Can you work these out from the model? Positions are in its coordinate system, mm. Round coordinates to 2 decimals unless told otherwise and drop trailing zeros. Loops run counter-clockwise (first coordinate to the right, second up) from the corner with the lowest first, then second, coordinate; pieces in that order, holes last.
(1) If I drill on line 1 along Z through (x, y) = (0, 0.3); line 2 along Y through (x, z) = (-25.5, 29), over which ranges is the centre line in solid material (lowest first)?
(2) I want a section at D-D on y = 10.75. Give the number of separate pieces and of enclosed holes in the cut face, plus the area to 3 significant figures.
(3) I want a section at C-C on y = 2.25. Write out the boundary of the cut face in (x, z), plus the area to 3 significant figures.
(4) I want a section at B-B on x = -6. Write out the boundary of the cut face in (y, z).
(5) Will these pins go through, and if not, where does the flat tip stop? pin 1 Ø0.8 at (x, z) = (33.5, 19) entering from +Y; pin 2 Ø4 at (x, y) = (30, 10) entering from -Z; pin 3 Ø11.5 at (x, z) = (27, -18.5) entering from +Y.
(6) I want a section at A-A on z = 0. Write out the boundary of the cut face in (x, y), plus the area to 3 significant figures.
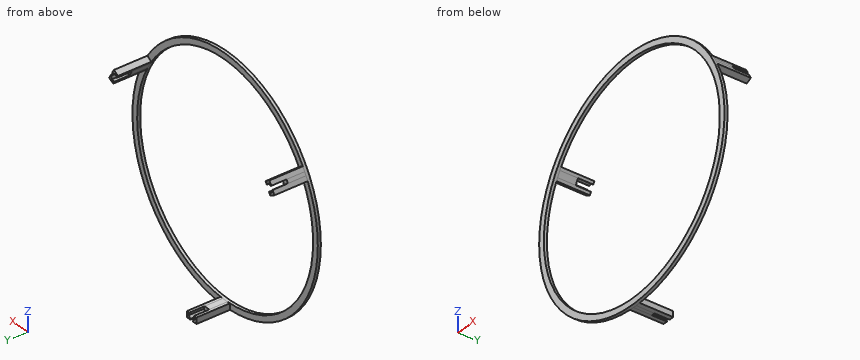
Autodesk Inventor part; units mm, degrees
ref_plane "YZ Plane" through (0, 0, 0) normal (1, 0, 0) x (0, 1, 0)
ref_plane "XZ Plane" through (0, 0, 0) normal (0, 1, 0) x (-1, 0, 0)
ref_plane "XY Plane" through (0, 0, 0) normal (0, 0, 1) x (1, 0, 0)
sketch "Sketch1" plane through (0, 0, 0) normal (0, 1, 0) x (-1, 0, 0)
  circle A0 centre (0, 0) radius 39.5
  circle A1 centre (0, 0) radius 37.5
  dimension "d0" = 79
  dimension "d1" = 75
extrude "Extrusion1" add sketch "Sketch1" along normal blind 1
sketch "Sketch2" plane through (0, 1, 0) normal (0, 1, 0) x (1, 0, 0)
  circle A0 centre (0, 0) radius 37.5
  circle A1 centre (0, 0) radius 39.5
  line L0 (0, 39.5) -> (0, 37.5) construction
  line L1 (-0.57, 39.24) -> (0, 39.24)
  line L2 (-1.31, 38.5) -> (-1.31, 38.5)
  line L3 (-1.31, 38.5) -> (-1.31, 38.49)
  line L4 (-1.2707, 37.74) -> (0, 37.74)
  line L5 (-0.57, 39.24) -> (-1.31, 38.5)
  line L6 (-1.31, 38.49) -> (-1.2707, 37.74)
  line L7 (0, 0) -> (2.0673, 39.4459) construction
  line L8 (0, 0) -> (-2.0673, 39.4459) construction
  line L9 (1.9626, 37.4486) -> (2.0673, 39.4459)
  line L10 (-1.9626, 37.4486) -> (-2.0673, 39.4459)
  line L11 (-1, 37.74) -> (-1, 37.4867)
  line L12 (0.57, 39.24) -> (0, 39.24)
  line L13 (1.31, 38.5) -> (1.31, 38.5)
  line L14 (1.31, 38.5) -> (1.31, 38.49)
  line L15 (1.2707, 37.74) -> (0, 37.74)
  line L16 (0.57, 39.24) -> (1.31, 38.5)
  line L17 (1.31, 38.49) -> (1.2707, 37.74)
  line L18 (-0.57, 39.24) -> (-0.57, 39.4959)
  line L19 (-0.57, 39.4959) -> (-2.0673, 39.4459)
  line L20 (-1, 37.4867) -> (-1.9646, 37.4867)
  line L21 (0.57, 39.24) -> (0.57, 39.4959)
  line L22 (0.57, 39.4959) -> (2.0673, 39.4459)
  line L23 (1, 37.4867) -> (1, 37.74)
  line L24 (1, 37.4867) -> (1.9646, 37.4867)
  line L25 (-33.6978, -20.1136) -> (-33.9828, -19.62)
  line L26 (-32.687, -20.3845) -> (-32.6783, -20.3795)
  line L27 (-32.0485, -19.9705) -> (-32.6838, -18.87)
  line L28 (-33.6978, -20.1136) -> (-32.687, -20.3845)
  line L29 (-32.6783, -20.3795) -> (-32.0485, -19.9705)
  line L30 (0, 0) -> (-33.1275, -21.5132) construction
  line L31 (-33.4127, -17.0246) -> (-35.1948, -17.9326)
  line L32 (-31.4501, -20.424) -> (-33.1275, -21.5132)
  line L33 (-32.1838, -19.736) -> (-31.9644, -19.6094)
  line L34 (-33.9883, -18.1105) -> (-33.3191, -17.7695)
  line L35 (-33.3191, -17.7695) -> (-32.6838, -18.87)
  line L36 (-34.2678, -19.1264) -> (-33.997, -18.1155)
  line L37 (-34.2678, -19.1264) -> (-33.9828, -19.62)
  line L38 (-33.997, -18.1155) -> (-33.9883, -18.1105)
  line L39 (-33.6978, -20.1136) -> (-33.9194, -20.2416)
  line L40 (-33.9194, -20.2416) -> (-33.1275, -21.5132)
  line L41 (-31.9644, -19.6094) -> (-31.4821, -20.4447)
  line L42 (-34.2678, -19.1264) -> (-34.4894, -19.2543)
  line L43 (-34.4894, -19.2543) -> (-35.1948, -17.9326)
  line L44 (-32.9644, -17.8773) -> (-33.1838, -18.004)
  line L45 (-32.9644, -17.8773) -> (-33.4467, -17.0419)
  line L46 (34.2678, -19.1264) -> (33.9828, -19.62)
  line L47 (33.997, -18.1155) -> (33.9883, -18.1105)
  line L48 (33.3191, -17.7695) -> (32.6838, -18.87)
  line L49 (34.2678, -19.1264) -> (33.997, -18.1155)
  line L50 (33.9883, -18.1105) -> (33.3191, -17.7695)
  line L51 (0, 0) -> (35.1948, -17.9326) construction
  line L52 (31.4501, -20.424) -> (33.1275, -21.5132)
  line L53 (33.4127, -17.0246) -> (35.1948, -17.9326)
  line L54 (33.1838, -18.004) -> (32.9644, -17.8773)
  line L55 (32.6783, -20.3795) -> (32.0485, -19.9705)
  line L56 (32.0485, -19.9705) -> (32.6838, -18.87)
  line L57 (33.6978, -20.1136) -> (32.687, -20.3845)
  line L58 (33.6978, -20.1136) -> (33.9828, -19.62)
  line L59 (32.687, -20.3845) -> (32.6783, -20.3795)
  line L60 (34.2678, -19.1264) -> (34.4894, -19.2543)
  line L61 (34.4894, -19.2543) -> (35.1948, -17.9326)
  line L62 (32.9644, -17.8773) -> (33.4467, -17.0419)
  line L63 (33.6978, -20.1136) -> (33.9194, -20.2416)
  line L64 (33.9194, -20.2416) -> (33.1275, -21.5132)
  line L65 (31.9644, -19.6094) -> (32.1838, -19.736)
  line L66 (31.9644, -19.6094) -> (31.4821, -20.4447)
  line L67 (-33.1838, -18.004) -> (-33.3191, -17.7695)
  line L68 (-33.3191, -17.7695) -> (-33.9883, -18.1105)
  line L69 (-33.997, -18.1155) -> (-33.9883, -18.1105)
  line L70 (-34.2678, -19.1264) -> (-33.997, -18.1155)
  line L71 (-33.6978, -20.1136) -> (-32.687, -20.3845)
  line L72 (-32.0485, -19.9705) -> (-32.6783, -20.3795)
  line L73 (-32.0485, -19.9705) -> (-32.1838, -19.736)
  line L74 (34.2678, -19.1264) -> (33.997, -18.1155)
  line L75 (33.1838, -18.004) -> (33.3191, -17.7695)
  line L76 (33.6978, -20.1136) -> (32.687, -20.3845)
  point P0 (-1.31, 39.24)
  point P1 (-1.31, 37.74)
  point P2 (0, 38.5)
  point P3 (1.31, 37.74)
  point P4 (-33.3278, -20.7545)
  point P5 (-32.0288, -20.0045)
  point P6 (-33.3388, -17.7355)
  point P7 (34.6378, -18.4855)
  point P8 (33.3388, -17.7355)
  point P9 (32.0288, -20.0045)
  dimension "d4" = 1.31
  dimension "d5" = 0.74
  dimension "d6" = 0.76
  dimension "d7" = 0.74
  dimension "d8" = 45
  dimension "d9" = 0.75
  dimension "d10" = 3
  dimension "d11" = 3
  dimension "d12" = 1
  dimension "d15" = 360
extrude "Extrusion2" add sketch "Sketch2" along normal blind 11 contours L23 L15 L17 L14 L16 L21 L22 L9 L24 | L62 L53 L61 L60 L49 L47 L50 L48 L54 | L20 L10 L19 L18 L5 L3 L6 L4 L11 | L65 L56 L55 L59 L57 L63 L64 L52 L66 | L44 L35 L34 L38 L36 L42 L43 L31 L45 | L41 L32 L40 L39 L28 L26 L29 L27 L33
sketch "Sketch3" plane through (0, 1, 0) normal (0, 1, 0) x (1, 0, 0)
  line L0 (33.1838, -18.004) -> (32.9644, -17.8773)
  arc A0 (31.9644, -19.6094) -> (32.9644, -17.8773) centre (0, 0) ccw
  line L1 (31.9644, -19.6094) -> (32.1838, -19.736)
  line L2 (32.1838, -19.736) -> (32.0485, -19.9705)
  line L3 (32.0485, -19.9705) -> (32.6783, -20.3795)
  line L4 (32.6783, -20.3795) -> (32.687, -20.3845)
  line L5 (32.687, -20.3845) -> (33.6978, -20.1136)
  line L6 (33.6978, -20.1136) -> (33.9194, -20.2416)
  arc A1 (33.9194, -20.2416) -> (34.4894, -19.2543) centre (0, 0) ccw
  line L7 (34.4894, -19.2543) -> (34.2678, -19.1264)
  line L8 (34.2678, -19.1264) -> (33.997, -18.1155)
  line L9 (33.997, -18.1155) -> (33.9883, -18.1105)
  line L10 (33.9883, -18.1105) -> (33.3191, -17.7695)
  line L11 (33.3191, -17.7695) -> (33.1838, -18.004)
extrude "Extrusion3" add sketch "Sketch3" along normal blind 6
sketch "Sketch4" plane through (0, 1, 0) normal (0, 1, 0) x (1, 0, 0)
  line L0 (-32.1838, -19.736) -> (-31.9644, -19.6094)
  arc A0 (-32.9644, -17.8773) -> (-31.9644, -19.6094) centre (0, 0) ccw
  line L1 (-32.9644, -17.8773) -> (-33.1838, -18.004)
  line L2 (-33.1838, -18.004) -> (-33.3191, -17.7695)
  line L3 (-33.3191, -17.7695) -> (-33.9883, -18.1105)
  line L4 (-33.9883, -18.1105) -> (-33.997, -18.1155)
  line L5 (-33.997, -18.1155) -> (-34.2678, -19.1264)
  line L6 (-34.2678, -19.1264) -> (-34.4894, -19.2543)
  arc A1 (-34.4894, -19.2543) -> (-33.9194, -20.2416) centre (0, 0) ccw
  line L7 (-33.9194, -20.2416) -> (-33.6978, -20.1136)
  line L8 (-33.6978, -20.1136) -> (-32.687, -20.3845)
  line L9 (-32.687, -20.3845) -> (-32.6783, -20.3795)
  line L10 (-32.6783, -20.3795) -> (-32.0485, -19.9705)
  line L11 (-32.0485, -19.9705) -> (-32.1838, -19.736)
extrude "Extrusion4" add sketch "Sketch4" along normal blind 6
sketch "Sketch5" plane through (0, 1, 0) normal (0, 1, 0) x (1, 0, 0)
  line L0 (-0.57, 39.4959) -> (-0.57, 39.24)
  line L1 (-0.57, 39.24) -> (-1.31, 38.5)
  line L2 (-1.31, 38.5) -> (-1.31, 38.49)
  line L3 (-1.31, 38.49) -> (-1.2707, 37.74)
  line L4 (-1.2707, 37.74) -> (-1, 37.74)
  line L5 (-1, 37.74) -> (-1, 37.4867)
  arc A0 (1, 37.4867) -> (-1, 37.4867) centre (0, 0) ccw
  line L6 (1, 37.4867) -> (1, 37.74)
  line L7 (1, 37.74) -> (1.2707, 37.74)
  line L8 (1.2707, 37.74) -> (1.31, 38.49)
  line L9 (1.31, 38.49) -> (1.31, 38.5)
  line L10 (1.31, 38.5) -> (0.57, 39.24)
  line L11 (0.57, 39.24) -> (0.57, 39.4959)
  arc A1 (0.57, 39.4959) -> (-0.57, 39.4959) centre (0, 0) ccw
extrude "Extrusion5" add sketch "Sketch5" along normal blind 6
properties part number "Hallhouder" material "ABS Plastic"
Filled sheet:
1. line 1: z = -39.5 to -37.5, 37.5 to 39.5
1. line 2: y = 0 to 1
2. separate pieces: 6
2. enclosed holes: 0
2. area: 11.6 mm2
3. outline: (-35.19, 17.93) - (-33.45, 17.04) - (-32.96, 17.88) arc R37.54 cw to (-31.96, 19.61) - (-31.48, 20.44) - (-33.13, 21.51) - (-33.92, 20.24) arc R39.58 ccw to (-34.49, 19.25) - close; (-2.07, -39.45) - (-0.57, -39.5) arc R39.5 ccw to (0.57, -39.5) - (2.07, -39.45) - (1.96, -37.49) - (1, -37.49) arc R37.5 cw to (-1, -37.49) - (-1.96, -37.49) - close; (31.48, 20.44) - (31.96, 19.61) arc R37.46 cw to (32.96, 17.88) - (33.45, 17.04) - (35.19, 17.93) - (34.49, 19.25) arc R39.42 ccw to (33.92, 20.24) - (33.13, 21.51) - close
3. area: 24.0 mm2
4. outline: (0, -39.04) - (1, -39.04) - (1, -37.02) - (0, -37.02) - close; (0, 37.02) - (1, 37.02) - (1, 39.04) - (0, 39.04) - close
5. pin 1: stops at y = 7
5. pin 2: stops at z = 19.61
5. pin 3: stops at y = 1
6. outline: (-39.5, 0) - (-37.5, 0) - (-37.5, 1) - (-39.5, 1) - close; (37.5, 0) - (39.5, 0) - (39.5, 1) - (37.5, 1) - close
6. area: 4.00 mm2
